Can you work these out from the model? Positions are in its coordinate system, mm. Give positions to 0.01 mm unless a question says otherwise; leave off trailing zeros. Loops run counter-clockwise (first coordinate to the right, second up) from the corner with the lowest first, then second, coordinate; pieces in that order, holes last. Notation, with made-up numbers: (-35, 48.25) - (-18, 48.25) arc R22 ccw to (-18, 56.25) - close; hole circle Ø11 at (49, 29). An arc over 180 degrees is marked (long way). Answer as a JSON object with one key per item and string values. Group by question number.
Item 1: Suppose I cut it at D-D on y = 126. Write out the boundary of the cut face in (x, z).
Item 2: Suppose I cut it at C-C on z = 0.85. Count the separate pieces of the cut face and the enclosed holes in it, and give its area (3 significant figures).
Item 3: Suppose I cut it at A-A on x = 107. Write out the boundary of the cut face in (y, z).
Item 4: Will these pins go through, and if not, where does the flat tip stop? pin 1 (3.5 mm diameter, centred on x = 99, y = 8, fed in from -Z); pin 2 (5 mm diameter, centred on x = 107, y = 126, fed in from -Z); pin 3 (6 mm diameter, centred on x = 34, y = 126, fed in from -Z).
Item 5: Suppose I cut it at B-B on y = 71. Write out the boundary of the cut face in (x, z), and give its area (3 significant figures).
Item 6: Thinking about a two-plate mould opening in Y: for faces 1 (the cylindrical face through (182.96, 55.33, 1.48)), 2 (the flat face through (102, 68, 3)), which applies, pulls with the +Y half, pulls with the -Y half, needs draft (parallel to the pull), parting line crosses it, or undercut?
Item 7: Please list where these lines run through material, in increasing order: L1, parallel to X at y = 35, z = 0.1; L2, parallel to X at y = 82, z = 2.85; L3, parallel to Y at x = 120.5, z = 1.
from build123d import *

# Parameters (mm, degrees)
SKETCH_1_W                 = 206
SKETCH_1_H                 = 134
SKETCH_1_R                 = 14
SKETCH_1_R_2               = 3.5
SKETCH_1_R_3               = 5.7
SKETCH_1_R_4               = 1
EXTRUDE_1_DEPTH            = 3
HOLE_WIZARD_M41_AT_2_COUNT = 2
HOLE_WIZARD_M41_AT_2_PITCH = 73
HOLE_WIZARD_M41_AT_3_COUNT = 2
HOLE_WIZARD_M41_AT_3_PITCH = 146
HOLE_WIZARD_M41_AT_4_COUNT = 2
HOLE_WIZARD_M41_AT_4_PITCH = 180.579622328
HOLE_WIZARD_M41_AT_5_COUNT = 2
HOLE_WIZARD_M41_AT_5_PITCH = 194.010309004
HOLE_WIZARD_M41_AT_6_COUNT = 2
HOLE_WIZARD_M41_AT_6_PITCH = 143.125818775
HOLE_WIZARD_M41_AT_7_COUNT = 2
HOLE_WIZARD_M41_AT_7_PITCH = 118.270875536
HOLE_WIZARD_M41_AT_8_COUNT = 2
HOLE_WIZARD_M41_AT_8_PITCH = 65.520989004


with BuildPart() as part:
    # Эскиз1 → Бобышка-Вытянуть1 (new body)
    with BuildSketch(Plane.XY):
        with Locations((103, 67)):
            Rectangle(SKETCH_1_W, SKETCH_1_H)
        with Locations((127.983323234, 74.939626383)):
            Circle(SKETCH_1_R, mode=Mode.SUBTRACT)
        with Locations((127.983323234, 35.24984102)):
            Circle(SKETCH_1_R, mode=Mode.SUBTRACT)
        with Locations((177.691125973, 35.560610723)):
            Circle(SKETCH_1_R_2, mode=Mode.SUBTRACT)
        with Locations((177.691125973, 24.371028973)):
            Circle(SKETCH_1_R_2, mode=Mode.SUBTRACT)
        with Locations((177.691125973, 79.434554566)):
            Circle(SKETCH_1_R_3, mode=Mode.SUBTRACT)
        with Locations((177.691125973, 57.509564132)):
            Circle(SKETCH_1_R_3, mode=Mode.SUBTRACT)
        with Locations((113.733323234, 89.189626383)):
            Circle(SKETCH_1_R_4, mode=Mode.SUBTRACT)
        with Locations((142.233323234, 89.189626383)):
            Circle(SKETCH_1_R_4, mode=Mode.SUBTRACT)
        with Locations((113.733323234, 49.49984102)):
            Circle(SKETCH_1_R_4, mode=Mode.SUBTRACT)
        with Locations((142.233323234, 49.49984102)):
            Circle(SKETCH_1_R_4, mode=Mode.SUBTRACT)
        with Locations((142.233323234, 20.99984102)):
            Circle(SKETCH_1_R_4, mode=Mode.SUBTRACT)
        with Locations((113.733323234, 20.99984102)):
            Circle(SKETCH_1_R_4, mode=Mode.SUBTRACT)
        with Locations((142.233323234, 60.689626383)):
            Circle(SKETCH_1_R_4, mode=Mode.SUBTRACT)
        with Locations((113.733323234, 60.689626383)):
            Circle(SKETCH_1_R_4, mode=Mode.SUBTRACT)
    extrude(amount=EXTRUDE_1_DEPTH)

    # Эскиз2 → Зенковка для винта с потайной головкой M41 (revolve, cut)
    with BuildSketch(Plane(origin=(26, 8, 0), x_dir=(0, 1, 0), z_dir=(1, 0, 0))):
        Polygon((0, 0), (0, 3), (2.4, 3), (2.25, 2.85), (2.25, 1.45), (3.7, 0), align=None)
    hole_wizard_m41 = revolve(axis=Axis((26, 8, -6.35), (0, 0, 1)), mode=Mode.SUBTRACT)

    # Зенковка для винта с потайной головкой M41 at 2: Зенковка для винта с потайной головкой M41 ×2
    with Locations(*[(i * HOLE_WIZARD_M41_AT_2_PITCH, 0, 0) for i in range(1, HOLE_WIZARD_M41_AT_2_COUNT)]):
        add(hole_wizard_m41, mode=Mode.SUBTRACT)

    # Зенковка для винта с потайной головкой M41 at 3: Зенковка для винта с потайной головкой M41 ×2
    with Locations(*[(i * HOLE_WIZARD_M41_AT_3_PITCH, 0, 0) for i in range(1, HOLE_WIZARD_M41_AT_3_COUNT)]):
        add(hole_wizard_m41, mode=Mode.SUBTRACT)

    # Зенковка для винта с потайной головкой M41 at 4: Зенковка для винта с потайной головкой M41 ×2
    with Locations(*[Vector(0.952488425, 0.304574787, 0) * (i * HOLE_WIZARD_M41_AT_4_PITCH) for i in range(1, HOLE_WIZARD_M41_AT_4_COUNT)]):
        add(hole_wizard_m41, mode=Mode.SUBTRACT)

    # Зенковка для винта с потайной головкой M41 at 5: Зенковка для винта с потайной головкой M41 ×2
    with Locations(*[Vector(0.793772253, 0.608215103, 0) * (i * HOLE_WIZARD_M41_AT_5_PITCH) for i in range(1, HOLE_WIZARD_M41_AT_5_COUNT)]):
        add(hole_wizard_m41, mode=Mode.SUBTRACT)

    # Зенковка для винта с потайной головкой M41 at 6: Зенковка для винта с потайной головкой M41 ×2
    with Locations(*[Vector(0.565935627, 0.824449432, 0) * (i * HOLE_WIZARD_M41_AT_6_PITCH) for i in range(1, HOLE_WIZARD_M41_AT_6_COUNT)]):
        add(hole_wizard_m41, mode=Mode.SUBTRACT)

    # Зенковка для винта с потайной головкой M41 at 7: Зенковка для винта с потайной головкой M41 ×2
    with Locations(*[Vector(0.067641336, 0.997709702, 0) * (i * HOLE_WIZARD_M41_AT_7_PITCH) for i in range(1, HOLE_WIZARD_M41_AT_7_COUNT)]):
        add(hole_wizard_m41, mode=Mode.SUBTRACT)

    # Зенковка для винта с потайной головкой M41 at 8: Зенковка для винта с потайной головкой M41 ×2
    with Locations(*[Vector(-0.274721128, 0.961523948, 0) * (i * HOLE_WIZARD_M41_AT_8_PITCH) for i in range(1, HOLE_WIZARD_M41_AT_8_COUNT)]):
        add(hole_wizard_m41, mode=Mode.SUBTRACT)


solid = part.part
Worked out:
{
 "1": {"outline": "(0, 0) - (30.3, 0) - (31.75, 1.45) - (31.75, 2.85) - (31.6, 3) - (0, 3) - close; (36.25, 1.45) - (37.7, 0) - (103.3, 0) - (104.75, 1.45) - (104.75, 2.85) - (104.6, 3) - (36.4, 3) - (36.25, 2.85) - close; (109.25, 1.45) - (110.7, 0) - (176.3, 0) - (177.75, 1.45) - (177.75, 2.85) - (177.6, 3) - (109.4, 3) - (109.25, 2.85) - close; (182.25, 1.45) - (183.7, 0) - (206, 0) - (206, 3) - (182.4, 3) - (182.25, 2.85) - close"},
 "2": {"separate pieces": "1", "enclosed holes": "22", "area": "25,900 mm2"},
 "3": {"outline": "(0, 0) - (122.3, 0) - (123.75, 1.45) - (123.75, 2.85) - (123.6, 3) - (0, 3) - close; (128.25, 1.45) - (129.7, 0) - (134, 0) - (134, 3) - (128.4, 3) - (128.25, 2.85) - close"},
 "4": {"pin 1": "passes through", "pin 2": "stops at z = 1.2", "pin 3": "stops at z = 0.7"},
 "5": {"outline": "(0, 0) - (4.3, 0) - (5.75, 1.45) - (5.75, 2.85) - (5.6, 3) - (0, 3) - close; (10.25, 1.45) - (11.7, 0) - (114.55, 0) - (114.55, 3) - (10.4, 3) - (10.25, 2.85) - close; (141.42, 0) - (206, 0) - (206, 3) - (141.42, 3) - close", "area": "522 mm2"},
 "6": {"face 1": "undercut", "face 2": "needs draft"},
 "7": {"L1": "x = 0 to 113.99, 141.98 to 174.24, 181.15 to 206", "L2": "x = 0 to 115.89, 140.07 to 172.6, 182.78 to 206", "L3": "y = 0 to 23.42, 47.08 to 63.11, 86.77 to 134"}
}
